```python
from build123d import *

# Parameters (mm, degrees)
BOSS_EXTRUDE1_DEPTH                  = 25.4
SKETCH4_W                            = 80
SKETCH4_H                            = 50
CUT_EXTRUDE1_DEPTH                   = 10
FILLET1_R                            = 5
F_12_0_12_DIAMETER_HOLE1_D           = 12
F_12_0_12_DIAMETER_HOLE1_CSINK_D     = 12.05
F_12_0_12_DIAMETER_HOLE1_CSINK_ANGLE = 100


with BuildPart() as part:
    # Sketch1 → Boss-Extrude1 (new body)
    with BuildSketch(Plane(origin=(0, 0, 0), x_dir=(1, 0, 0), z_dir=(0, 1, 0))):
        with BuildLine():
            Line((-140, 75), (140, 75))
            ThreePointArc((140, 75), (147.071067812, 72.071067812), (150, 65))
            Line((150, 65), (150, -65))
            ThreePointArc((150, -65), (147.071067812, -72.071067812), (140, -75))
            Line((140, -75), (-140, -75))
            ThreePointArc((-140, -75), (-147.071067812, -72.071067812), (-150, -65))
            Line((-150, -65), (-150, 65))
            ThreePointArc((-150, 65), (-147.071067812, 72.071067812), (-140, 75))
        make_face()
    extrude(amount=BOSS_EXTRUDE1_DEPTH)

    # Sketch4 → Cut-Extrude1 (cut)
    with BuildSketch(Plane(origin=(0, 25.4, 0), x_dir=(1, 0, 0), z_dir=(0, 1, 0))):
        Rectangle(SKETCH4_W, SKETCH4_H)
    extrude(amount=-CUT_EXTRUDE1_DEPTH, mode=Mode.SUBTRACT)

    # Fillet1
    fillet1_edges = [part.edges().sort_by_distance(p)[0] for p in [
        (40, 20.4, -25),
        (40, 20.4, 25),
        (-40, 20.4, 25),
        (-40, 20.4, -25),
    ]]
    fillet(fillet1_edges, radius=FILLET1_R)

    # Ø12.0 (12) Diameter Hole1 (through all)
    with Locations(Plane(origin=(0, 25.4, 0), x_dir=(1, 0, 0), z_dir=(0, 1, 0))):
        with Locations((-125, 50), (125, 50), (125, -50), (-125, -50)):
            CounterSinkHole(F_12_0_12_DIAMETER_HOLE1_D / 2, F_12_0_12_DIAMETER_HOLE1_CSINK_D / 2, counter_sink_angle=F_12_0_12_DIAMETER_HOLE1_CSINK_ANGLE)


solid = part.part
```
The model under review builds one solid part; all positions refer to its coordinate system, in mm. Round coordinates to 2 decimals unless told otherwise and drop trailing zeros. Write each loop counter-clockwise with the first axis right and the second up, starting at its lowest first coordinate (ties: lowest second). Pieces come first, ordered by that corner, then holes.
(1) Mouldability with a two-part tool opening along X and no side actions: class faces 1 (the flat face through (40, 20, 0)), 2 (the flat face through (2, 25.4, 32)), 3 (the flat face through (150, 13, -1)), 4 (the flat face through (0, 20, -25)) as +X half, -X half, draft (parallel to the pull), parting line (faces both ways), or undercut.
(2) We need section C-C on x = 125. Give the boundary of the cut face in (y, z) (3 decimals).
(3) Wall thickness on L1, parallel to X at y = 20.5, z = -50; L2, parallel to Z at x = 125, y = 7.5; L3, parallel to X at y = 21.25, z = 14: over which ranges is each line inside the solid? List them lowest first.
(4) Insertion check: pin 1 (7 mm diameter, centred on x = -125, z = 50, fed in from +Y). The pin has a flat end and moves straight along its axis. Give the tip position at first contact, or say it passes through.
(5) We need section A-A on y = 22. Give the boundary of the cut face in (x, z).
(6) We need section D-D on z = 13.5. Give the boundary of the cut face in (x, y).
(7) We need section B-B on z = 50. Give the boundary of the cut face in (x, y) (3 decimals), and give its area (3 significant figures).
Findings below:
1. face 1: undercut
1. face 2: draft
1. face 3: +X half
1. face 4: undercut
2. outline: (0, -75) - (25.4, -75) - (25.4, -56.025) - (25.379, -56) - (0, -56) - close; (0, -44) - (25.379, -44) - (25.4, -43.975) - (25.4, 43.975) - (25.379, 44) - (0, 44) - close; (0, 56) - (25.379, 56) - (25.4, 56.025) - (25.4, 75) - (0, 75) - close
3. L1: x = -150 to -131, -119 to 119, 131 to 150
3. L2: z = -75 to -56, -44 to 44, 56 to 75
3. L3: x = -150 to -40, 40 to 150
4. pin 1: passes through
5. outline: (-150, -65) arc R10 ccw to (-140, -75) - (140, -75) arc R10 ccw to (150, -65) - (150, 65) arc R10 ccw to (140, 75) - (-140, 75) arc R10 ccw to (-150, 65) - close; hole circle Ø12 at (-125, -50); hole circle Ø12 at (-125, 50); hole (-40, -20) arc R5 ccw to (-35, -25) - (35, -25) arc R5 ccw to (40, -20) - (40, 20) arc R5 ccw to (35, 25) - (-35, 25) arc R5 ccw to (-40, 20) - close; hole circle Ø12 at (125, -50); hole circle Ø12 at (125, 50)
6. outline: (-150, 0) - (150, 0) - (150, 25.4) - (40, 25.4) - (40, 15.4) - (-40, 15.4) - (-40, 25.4) - (-150, 25.4) - close
7. outline: (-150, 0) - (-131, 0) - (-131, 25.379) - (-131.025, 25.4) - (-150, 25.4) - close; (-119, 0) - (119, 0) - (119, 25.379) - (118.975, 25.4) - (-118.975, 25.4) - (-119, 25.379) - close; (131, 0) - (150, 0) - (150, 25.4) - (131.025, 25.4) - (131, 25.379) - close
7. area: 7,010 mm2
